Job drawing, mm, ordinate dimensions from the low corner. One solid piece. A direction names the side the tool comes from. Round coordinates to 2 decimals unless told otherwise and drop trailing zeros. Write each loop counter-clockwise with the first axis right and the second up, starting at its lowest first coordinate (ties: lowest second). Pieces come first, ordered by that corner, then holes. Notation, with made-up numbers: M 69,-21 L 124,-21 A24 cw 124,1 Z; hole C 54.25,25.25 d3. An arc over 180 degrees is marked long. Write each question's results on one line, items separated by ' | '. Start each with the question number.
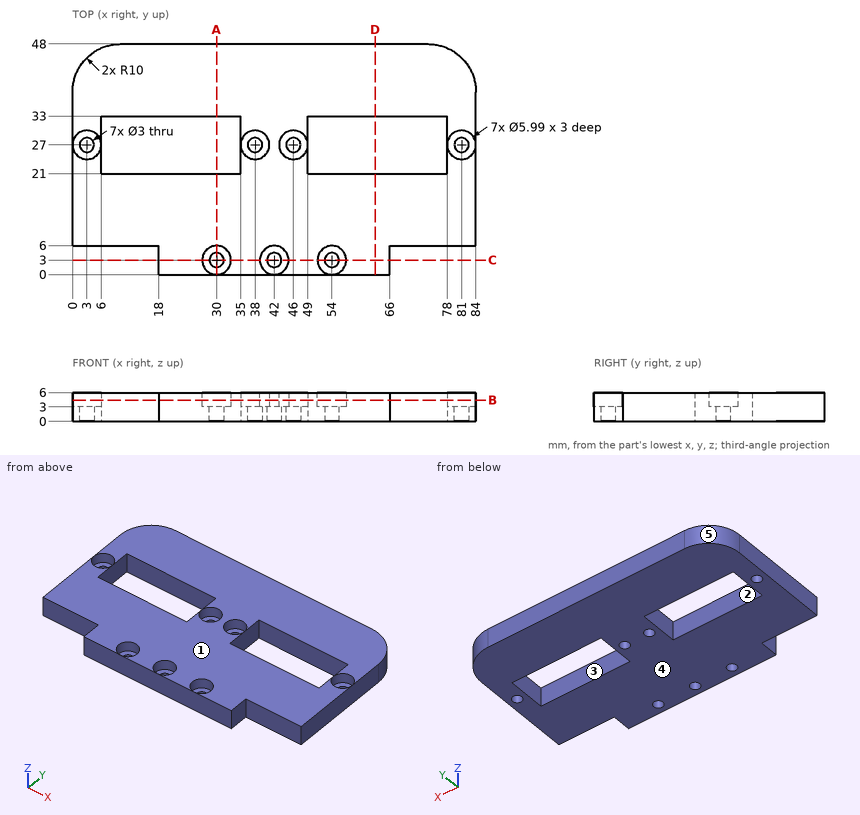
1) Wall check: line 1 along Y through (x, z) = (38, 2.8); line 2 along Y through (x, z) = (64, 3.3); line 3 along Y through (x, z) = (40.5, 4.85). Give the ranges that are in metal, low to high. Write a range as from..to.
2) Saw through at A-A, the plane x = 30. Write the cut outline in (y, z) (3 decimals).
3) Drop flat-ended pins along their axis: pin 1 Ø1 at (x, y) = (56.5, 20.5) entering from -Z; pin 2 Ø3.5 at (x, y) = (30, 3) entering from +Z. Give the stop position or say it passes through.
4) Saw through at D-D, the plane x = 63. Write the cut outline in (y, z), plus the area to 3 significant figures.
5) Saw through at C-C, the plane y = 3. Write the cut outline in (x, z) (3 decimals), plus the area to 3 significant figures.
6) Pull direction X, two halves, no side cores. Call the marked faces 3, 4 and 5: pulls with the +X half, pulls with the -X half, needs draft (parallel to the pull), parting line crosses it, or undercut.
7) 3-axis set-ups, long thin cutter, end or side, ignore diameter. For the marked faces 1 and 2: which of +Z, -Z, +X, -X, +Y, -Y reach the whole face in a straight line?
8) Saw through at B-B, the plane z = 4.4. State how many separate pieces and enclosed holes the cut face has, plus the area to 3 significant figures.
Filled sheet:
1) line 1: y = 0..25.5, 28.5..48 | line 2: y = 0..21, 33..48 | line 3: y = 0..0.41, 5.59..25.35, 28.65..48
2) outline: M 0,0 L 1.5,0 L 1.5,3 L 0.005,3 L 0.005,6 L 0,6 Z; M 4.5,0 L 21,0 L 21,6 L 5.995,6 L 5.995,3 L 4.5,3 Z; M 33,0 L 48,0 L 48,6 L 33,6 Z
3) pin 1: stops at z = 0 | pin 2: stops at z = 3
4) outline: M 0,0 L 21,0 L 21,6 L 0,6 Z; M 33,0 L 48,0 L 48,6 L 33,6 Z | area: 216 mm^2
5) outline: M 18,0 L 28.5,0 L 28.5,3 L 27.005,3 L 27.005,6 L 18,6 Z; M 31.5,0 L 40.5,0 L 40.5,3 L 39.005,3 L 39.005,6 L 32.995,6 L 32.995,3 L 31.5,3 Z; M 43.5,0 L 52.5,0 L 52.5,3 L 51.005,3 L 51.005,6 L 44.995,6 L 44.995,3 L 43.5,3 Z; M 55.5,0 L 66,0 L 66,6 L 56.995,6 L 56.995,3 L 55.5,3 Z | area: 207 mm^2
6) face 3: undercut | face 4: needs draft | face 5: pulls with the -X half
7) face 1: +Z, +X, -X, +Y, -Y | face 2: +Z, -Z
8) separate pieces: 1 | enclosed holes: 9 | area: 2,880 mm^2
